```python
from build123d import *

# Parameters (mm, degrees)
F0_W     = 20
F0_H     = 40
F1_DEPTH = 20
F2_W     = 15
F2_H     = 15
F2_R     = 2.5
F3_DEPTH = 20.001
F4_W     = 15
F4_H     = 15
F4_R     = 2.5
F5_DEPTH = 20.001
F6_R     = 2.5
F7_DEPTH = 40.001


with BuildPart() as f1:
    # F0 (on Front) → F1 (new body)
    with BuildSketch(Plane.XZ):
        Rectangle(F0_W, F0_H)
    extrude(amount=F1_DEPTH)

    # F2 (on face) → F3 (cut, through all)
    with BuildSketch(Plane.YZ.offset(10)):
        with Locations((-10, 10)):
            Rectangle(F2_W, F2_H)
        with Locations((-10, -10)):
            Circle(F2_R)
    extrude(amount=-F3_DEPTH, mode=Mode.SUBTRACT)

    # F4 (on face) → F5 (cut, through all)
    with BuildSketch(Plane(origin=(0, 0, 0), x_dir=(-1, 0, 0), z_dir=(0, 1, 0))):
        with Locations((0, -10)):
            Rectangle(F4_W, F4_H)
        with Locations((0, 10)):
            Circle(F4_R)
    extrude(amount=-F5_DEPTH, mode=Mode.SUBTRACT)

    # F6 (on face) → F7 (cut, through all)
    with BuildSketch(Plane.XY.offset(20)):
        with Locations((0, -10)):
            Circle(F6_R)
    extrude(amount=-F7_DEPTH, mode=Mode.SUBTRACT)


solid = f1.part
```
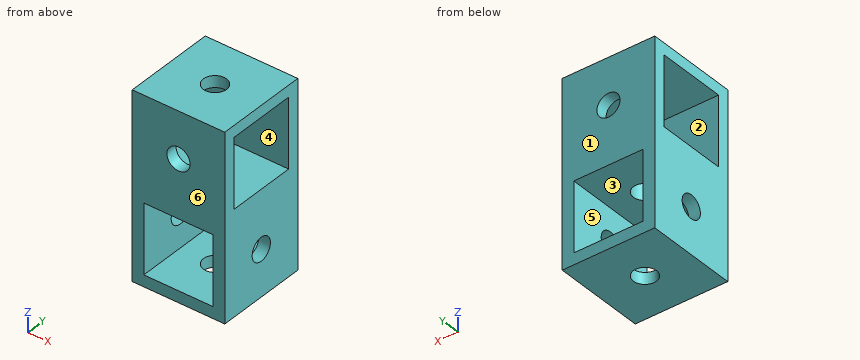
Could you check a few things on this model? Use its own coordinates, in mm. Face numbers are marked on the shaded views. A direction names the side the tool comes from. Round coordinates to 2 decimals unless told otherwise and drop trailing zeros. Write each loop counter-clockwise with the first axis right and the second up, starting at its lowest first coordinate (ties: lowest second). Pieces come first, ordered by that corner, then holes. Notation, with made-up numbers: M -38.75,35.5 L -34.75,35.5 A36 cw -34.75,70.5 Z; hole C 2,27.5 d7. An arc over 180 degrees is marked long. Answer in a Markdown table with one row per item. Add a question column.
Q1. Imagine slicing it at B-B (z = 10). Please give me the cut outline in (x, y).
Q2. Imagine slicing it at A-A (y = -10). Give the number of separate pieces and of enclosed holes in the cut face, then the cut area to 3 significant figures.
Q3. If we mould it in two halves opening along Y, with no side actions, what happens to the marked faces 1, 2 and 3? For each: +Y half, -Y half, draft (parallel to the pull), parting line (faces both ways), or undercut.
Q4. If I drill on line 1 (Z direction, x = -5.5, y = -8.5); line 2 (Z direction, x = 0, y = -19.25); line 3 (Y direction, x = 3.5, z = 13), over which ranges is the centre line in solid material (lowest first)? Write a range as from..to.
Q5. Imagine slicing it at D-D (y = -14). Please give me the cut outline in (x, z).
Q6. On a 3-axis mill with a long thin cutter (end or side, diameter ignored), from which of +Z, -Z, +X, -X, +Y, -Y can I reach the whole of each face in a straight line? I mean the marked faces 4, 5 and 6. Say none if no direction works.
Values:
| question | item | result |
|---|---|---|
| 1 | outline | M -10,-20 L -2.5,-20 L -2.5,-17.5 L -10,-17.5 Z; M -10,-2.5 L -2.5,-2.5 L -2.5,0 L -10,0 Z; M 2.5,-20 L 10,-20 L 10,-17.5 L 2.5,-17.5 Z; M 2.5,-2.5 L 10,-2.5 L 10,0 L 2.5,0 Z |
| 2 | separate pieces | 6 |
| 2 | enclosed holes | 0 |
| 2 | area | 200 mm^2 |
| 3 | face 1 | +Y half |
| 3 | face 2 | undercut |
| 3 | face 3 | draft |
| 4 | line 1 | -20..-17.5, -2.5..2.5, 17.5..20 |
| 4 | line 2 | -20..-17.5, -2.5..7.5, 12.5..20 |
| 4 | line 3 | -20..-17.5, -2.5..0 |
| 5 | outline | M -10,-20 L 10,-20 L 10,2.5 L -10,2.5 Z; M -10,17.5 L 10,17.5 L 10,20 L -10,20 Z; hole M -7.5,-17.5 L 7.5,-17.5 L 7.5,-2.5 L -7.5,-2.5 Z |
| 6 | face 4 | +X, -X |
| 6 | face 5 | +Y, -Y |
| 6 | face 6 | +Z, -Z, +X, -X, -Y |
